Geometry: final body of the model. Coordinates: model frame, mm. A direction names the side the tool comes from. Round coordinates to 2 decimals unless told otherwise and drop trailing zeros. Order: outer loops, then holes, each group sorted by start corner. A loop starts at its lowest first (then second) coordinate and runs counter-clockwise, first axis right, second up. Notation, with made-up numbers: M -9,38 L 13,38 A24 cw 13,74 Z; hole C 78.5,-16.5 d3. An arc over 180 degrees is marked long. Return JSON: item names as keys, results as strings. Group by question number.
Q1. Cut plane B-B on y = -1.5. Output: boundary loops of the cut face in (x, z), and give its area (3 significant figures).
Q2. Ray query, probe 1 along Y at (x, z) = (22, 5); probe 2 along Z at (x, y) = (-22, -3.75); probe 3 along Y at (x, z) = (58, 2). Return the intervals inside material, ascending.
Q3. Contact query for flat-ended pins moving along their axis: pin 1 (2 mm diameter, centred on x = -29, y = -1.5, fed in from +Z); pin 2 (10 mm diameter, centred on x = -20, z = 10, fed in from -Y); pin 3 (4 mm diameter, centred on y = 1.5, z = 7, fed in from +X); pin 4 (12 mm diameter, centred on x = -16.5, z = 10, fed in from -Y). Output: stop coordinate, or through.
Q4. Access query for faces 1 (the face through (-1, 0, 0)), 2 (the face through (-0.9, 3.9, 1.8)). Directions: +Z, -Z, +X, -X, +Y, -Y. A direction counts if a zero-diameter tool reaches every point of the face in a straight line with its end or side. Return the directions, or none.
Q5. Cut plane C-C on z = 9.5. Output: boundary loops of the cut face in (x, y).
Q6. Mould query, pull axis Y, two halves, no side actions, for faces 3 (the face through (-1, -4.9, 3)), 4 (the face through (65, 5.3, 4.2)), 5 (the face through (-1, 5.5, 10)). Classes: released by +Y, released by -Y, zero draft, split by the parting line, or undercut.
```python
from build123d import *

# Parameters (mm, degrees)
SKETCH_1_W      = 130
SKETCH_1_H      = 11
EXTRUDE_1_DEPTH = 0.8
SKETCH_2_W      = 130
SKETCH_2_H      = 0.6
EXTRUDE_2_DEPTH = 20
SKETCH_3_W      = 130
SKETCH_3_H      = 2
EXTRUDE_3_DEPTH = 2
CHAMFER_1_SIZE  = 2
SKETCH_4_W      = 130
SKETCH_4_H      = 0.6
EXTRUDE_4_DEPTH = 4
SKETCH_5_W      = 130
SKETCH_5_H      = 0.8
EXTRUDE_5_DEPTH = 0.8
CHAMFER_2_SIZE  = 0.8


with BuildPart() as part:
    # 草图1 → 凸台-拉伸1 (new body)
    with BuildSketch(Plane.XY):
        Rectangle(SKETCH_1_W, SKETCH_1_H)
    extrude(amount=EXTRUDE_1_DEPTH)

    # 草图2 → 凸台-拉伸2 (add)
    with BuildSketch(Plane.XY.offset(0.8)):
        with Locations((0, 5.2)):
            Rectangle(SKETCH_2_W, SKETCH_2_H)
    extrude(amount=EXTRUDE_2_DEPTH)

    # 草图3 → 凸台-拉伸3 (add)
    with BuildSketch(Plane.XY.offset(0.8)):
        with Locations((0, 3.9)):
            Rectangle(SKETCH_3_W, SKETCH_3_H)
    extrude(amount=EXTRUDE_3_DEPTH)

    # 倒角1
    chamfer_1_edges = [part.edges().sort_by_distance(p)[0] for p in [
        (0, 2.9, 2.8),
    ]]
    chamfer(chamfer_1_edges, length=CHAMFER_1_SIZE - 0.0001)  # a hair under: the kernel refuses the full size

    # 草图4 → 凸台-拉伸4 (add)
    with BuildSketch(Plane.XY.offset(0.8)):
        with Locations((0, -5.2)):
            Rectangle(SKETCH_4_W, SKETCH_4_H)
    extrude(amount=EXTRUDE_4_DEPTH)

    # 草图5 → 凸台-拉伸5 (add)
    with BuildSketch(Plane.XY.offset(0.8)):
        with Locations((0, -4.5)):
            Rectangle(SKETCH_5_W, SKETCH_5_H)
    extrude(amount=EXTRUDE_5_DEPTH)

    # 倒角2
    chamfer_2_edges = [part.edges().sort_by_distance(p)[0] for p in [
        (0, -4.1, 1.6),
    ]]
    chamfer(chamfer_2_edges, length=CHAMFER_2_SIZE - 0.0001)  # a hair under: the kernel refuses the full size


solid = part.part
```
Result sheet:
{
 "1": {"outline": "M -65,0 L 65,0 L 65,0.8 L -65,0.8 Z", "area": "104 mm²"},
 "2": {"probe 1": "y = 4.9 to 5.5", "probe 2": "z = 0 to 0.8", "probe 3": "y = -5.5 to -4.9, 4.1 to 5.5"},
 "3": {"pin 1": "stops at z = 0.8", "pin 2": "stops at y = 4.9", "pin 3": "passes through", "pin 4": "stops at y = -5.5"},
 "4": {"face 1": "-Z, +X, -X, +Y, -Y", "face 2": "+Z, +X, -X"},
 "5": {"outline": "M -65,4.9 L 65,4.9 L 65,5.5 L -65,5.5 Z"},
 "6": {"face 3": "undercut", "face 4": "zero draft", "face 5": "released by +Y"}
}
